Can you work these out from the model? Positions are in its coordinate system, mm. A direction names the side the tool comes from. Give positions to 0.01 mm unless a question says otherwise; leave off trailing zeros. Order: outer loops, then holes, each group sorted by start corner. A loop starts at its lowest first (then second) coordinate and runs counter-clockwise, first axis right, second up. Notation, with made-up numbers: M 70.25,61 L 115.25,61 A21 ccw 115.25,76 Z; hole C 8.25,-2.5 d1. An arc over 180 degrees is marked long. Use a Markdown table: item, result. Add a question column.
Autodesk Fusion 360 part; units mm, degrees
sketch "Sketch1" plane through (0, 0, 0) normal (0, 0, 1) x (1, 0, 0)
  line L0 (10, -7) -> (-10, -7)
  line L1 (-10, 7) -> (10, 7)
  line L2 (5, 7) -> (-5, -7) construction
  line L3 (5, -7) -> (-5, 7) construction
  line L4 (10, 0) -> (-10, 0) construction
  line L5 (0, -9.75) -> (0, 9.75) construction
  circle A0 centre (0, -9.75) radius 1.5
  circle A1 centre (0, 9.75) radius 1.5
  line L6 (-10, -15.75) -> (10, -15.75)
  line L7 (-10, 15.75) -> (10, 15.75)
  line L8 (-10, -15.75) -> (-10, 15.75)
  line L9 (10, -15.75) -> (10, 15.75)
  dimension "d1" = 14
  dimension "d2" = 10
  dimension "d3" = 3
  dimension "d4" = 3
  dimension "d5" = 19.5
  dimension "d6" = 20
extrude "Extrude1" add sketch "Sketch1" along normal blind 20 contours L0 L6 L8 L9 | L1 L7 L8 L9 makes body 1 at (-3.3333, -15.75, 6.6667) makes body 2 at (-3.3333, 7, 6.6667)
extrude "Extrude2" add sketch "Sketch1" along normal blind 16 contours L0 L1 L8 L9 bodies 1 2
sketch "Sketch2" plane through (0, -15.75, 0) normal (0, -1, 0) x (1, 0, 0)
  line L0 (-10, 0) -> (10, 0)
  line L1 (10, 0) -> (10, 20)
  line L2 (10, 20) -> (-10, 20)
  line L3 (-10, 20) -> (-10, 0)
  circle A0 centre (0, 9.8899) radius 2.65
  dimension "d11" = 5.3
extrude "Extrude3" add sketch "Sketch1" along normal blind 14 contours A0 | A1 bodies 1
extrude "Extrude4" cut sketch "Sketch2" against normal blind 31.5 contours A0 bodies 1
sketch "Sketch3" plane through (0, 0, 0) normal (0, 0, 1) x (1, 0, 0)
  line L0 (-10, -15.75) -> (-10, 15.75)
  line L1 (10, -15.75) -> (10, 15.75)
  line L2 (-2.9, -17.25) -> (2.9, -17.25)
  line L3 (2.9, -15.75) -> (2.9, -17.25)
  line L4 (-2.9, -15.75) -> (-2.9, -17.25)
  line L5 (-10, -15.75) -> (-2.9, -15.75)
  line L6 (2.9, -15.75) -> (10, -15.75)
  line L7 (-2.9, -15.75) -> (2.9, -15.75)
  line L8 (-10, -15.75) -> (10, -15.75)
  line L9 (0, 0) -> (0, -34.5) construction
  dimension "d23" = 1.5
  dimension "d27" = 5.8
extrude "Extrude5" add sketch "Sketch3" along normal blind 20 bodies 1
extrude "Extrude6" cut sketch "Sketch2" along normal blind 3 contours A0 bodies 1
chamfer "Chamfer1" distance 1.5 angle 45 1 edges at (2.9, -15.75, 10) on bodies 1
chamfer "Chamfer1" distance 1.5 angle 45 1 edges at (-2.9, -15.75, 10) on bodies 1
sketch "Sketch4" plane through (0, 15.75, 0) normal (0, 1, 0) x (-1, 0, 0)
  circle A0 centre (0, 9.8899) radius 2.65
  line L0 (-10, 0) -> (10, 0)
  line L1 (10, 0) -> (10, 20)
  line L2 (10, 20) -> (-10, 20)
  line L3 (-10, 20) -> (-10, 0)
  circle A1 centre (0, 9.8899) radius 5
  dimension "d24" = 10
extrude "Extrude7" cut sketch "Sketch4" against normal blind 5 contours A1 bodies 1
sketch "Sketch5" plane through (0, 0, 0) normal (0, 0, 1) x (1, 0, 0)
  line L0 (2.65, -17.25) -> (-2.65, -17.25)
  line L1 (2.65, -17.25) -> (-2.65, -17.25)
sketch "Sketch6" plane through (0, -15.75, 0) normal (0, -1, 0) x (1, 0, 0)
  line L0 (4.7787, 4.9544) -> (-4.7787, 4.9544)
  line L1 (-4.7787, 4.9544) -> (-4.7787, 16.3254)
  line L2 (-4.7787, 16.3254) -> (4.7787, 16.3254)
  line L3 (4.7787, 16.3254) -> (4.7787, 4.9544)
  point P0 (0, 9.8899)
  point P1 (0, 9.8899)
extrude "Extrude8" cut sketch "Sketch6" along normal blind 1.5 bodies 1
chamfer "Chamfer2" distance 1.5 angle 45 1 edges at (0, -15.75, 16.3254) on bodies 1
chamfer "Chamfer3" distance 1.5 angle 45 1 edges at (0, -17.25, 4.9544) on bodies 1
1. If we section it at B-B, the plane z = 11.5: List the corners of the cut face in (x, y) for me, then the cut area to 3 significant figures.
2. If we section it at D-D, the plane x = -7: List the corners of the cut face in (y, z) for me.
3. Will these pins go through, and if not, where does the flat tip stop? pin 1 (3 mm diameter, centred on x = 1.5, z = 11, fed in from +Y); pin 2 (7 mm diameter, centred on x = 0, y = -1, fed in from +Z); pin 3 (1.5 mm diameter, centred on x = 0.5, y = -9.5, fed in from +Z).
4. On a 3-axis mill with a long thin cutter (end or side, diameter ignored), from which of +Z, -Z, +X, -X, +Y, -Y can I reach the whole of each face in a straight line? I mean faces 4 (the face through (-2.307, 13.285, 5.454)), 5 (the face through (-0.325, -8.286, 16.958)), 6 (the face through (0, 7, 18)), 7 (the face through (0.062, -16.511, 4.194)). Say none if no direction works.
5. If we section it at C-C, the plane y = -9.75: List the corners of the cut face in (x, z) for me, then the cut area to 3 significant figures.
6. We'd pull the mould along Z, two halves only. Please class faces 1 (the face through (3.66, -16.49, 18.02)), 2 (the face through (0, -10, 14)), 3 (the face through (0.062, -16.51, 15.586)): +Z half, -Z half, draft (parallel to the pull), parting line (faces both ways), or undercut.
7. If we section it at A-A, the plane x = 0: State how many separate pieces and enclosed holes the cut face has, then the cut area to 3 significant figures.
8. I need wall thicknesses on L1, parallel to Y at x = 0, z = 17; L2, parallel to X at y = 9.75, z = 16.75; L3, parallel to Y at x = -6, z = 16.25. Which ranges of each line are inside material? Lowest first, please. Write a range as [from, to].
Geometry results:
| question | item | result |
|---|---|---|
| 1 | outline | M -10,-15.75 L -2.1,-15.75 L -2.1,10.75 L -4.73,10.75 L -4.73,15.75 L -10,15.75 Z; M 2.1,-15.75 L 10,-15.75 L 10,15.75 L 4.73,15.75 L 4.73,10.75 L 2.1,10.75 Z |
| 1 | area | 471 mm^2 |
| 2 | outline | M -15.75,0 L 15.75,0 L 15.75,20 L 7,20 L 7,16 L -7,16 L -7,20 L -15.75,20 Z |
| 3 | pin 1 | stops at y = 10.75 |
| 3 | pin 2 | stops at z = 16 |
| 3 | pin 3 | stops at z = 14 |
| 4 | face 4 | +Y |
| 4 | face 5 | +Z |
| 4 | face 6 | +Z, +X, -X |
| 4 | face 7 | +X, -X, -Y |
| 5 | outline | M -10,0 L 10,0 L 10,20 L 1.5,20 L 1.5,14 L -1.5,14 L -1.5,20 L -10,20 Z; hole C 0,9.89 d5.3 |
| 5 | area | 360 mm^2 |
| 6 | face 1 | draft |
| 6 | face 2 | +Z half |
| 6 | face 3 | undercut |
| 7 | separate pieces | 3 |
| 7 | enclosed holes | 0 |
| 7 | area | 361 mm^2 |
| 8 | L1 | y = [-17.25, -11.25], [-8.25, -7], [7, 8.25], [11.25, 15.75] |
| 8 | L2 | x = [-10, -1.5], [1.5, 10] |
| 8 | L3 | y = [-15.75, -7], [7, 15.75] |
